```python
from build123d import *

# Parameters (mm, degrees)
F1_DEPTH = 2


with BuildPart() as f1:
    # F0 (on Top) → F1 (new body)
    with BuildSketch(Plane.XY):
        with BuildLine():
            Line((12, 38), (0, 38))
            Line((0, 38), (-12, 38))
            ThreePointArc((-12, 38), (-19.071081, 35.071055), (-22, 27.999963))
            Line((-22, 27.999963), (-22, 21.999963))
            ThreePointArc((-22, 21.999963), (-23.171507, 19.171602), (-25.999815, 17.999963))
            Line((-25.999815, 17.999963), (-28.499815, 17.999963))
            Line((-28.499815, 17.999963), (-28.499815, -7.000037))
            Line((-28.499815, -7.000037), (-25.999815, -7.000037))
            ThreePointArc((-25.999815, -7.000037), (-9.507625, -19.877017), (-18, -39))
            Line((-18, -39), (-18, -42))
            Line((-18, -42), (0, -42))
            Line((0, -42), (18, -42))
            Line((18, -42), (18, -39))
            ThreePointArc((18, -39), (9.507625, -19.877017), (25.999815, -7.000037))
            Line((25.999815, -7.000037), (28.499815, -7.000037))
            Line((28.499815, -7.000037), (28.499815, 17.999963))
            Line((28.499815, 17.999963), (25.999815, 17.999963))
            ThreePointArc((25.999815, 17.999963), (23.171507, 19.171602), (22, 21.999963))
            Line((22, 21.999963), (22, 27.999963))
            ThreePointArc((22, 27.999963), (19.071081, 35.071055), (12, 38))
        make_face()
    extrude(amount=F1_DEPTH)


solid = f1.part
```
Read the model definition and answer for the solid it produces. Units are mm, in the model's axes. A direction names the side the tool comes from. Coordinates: 2 decimals unless noted, no trailing zeros. Write each loop counter-clockwise with the first axis right and the second up, starting at its lowest first coordinate (ties: lowest second). Pieces come first, ordered by that corner, then holes. Notation, with made-up numbers: (50.25, 62) -> (96.25, 62) arc R22 ccw to (96.25, 98) -> close; hole circle Ø3 at (88, 89). An arc over 180 degrees is marked (long way). Return JSON: item names as keys, results as strings.
1. A cutting plane is placed at D-D (x = 10). Determine the outline of the cut face in (y, z).
Found:
{"outline": "(-42, 0) -> (-29.74, 0) -> (-29.74, 2) -> (-42, 2) -> close; (-18.26, 0) -> (38, 0) -> (38, 2) -> (-18.26, 2) -> close"}
2. A cutting plane is placed at C-C (y = -22). Determine the outline of the cut face in (x, z), and give its area (3 significant figures).
Found:
{"outline": "(-9.12, 0) -> (9.12, 0) -> (9.12, 2) -> (-9.12, 2) -> close", "area": "36.5 mm2"}
3. Each of these flat-tipped pins is pushed along its axis until it touches: P1, Ø1, axis at x = -27.5, z = 1, coming from the -Y side; P2, Ø1, axis at y = 24, z = 0.5, coming from the +X side; P3, Ø0.6, axis at y = -41, z = 1, coming from the -X side. Where does it stop, or does it pass through?
Found:
{"P1": "y = -7", "P2": "x = 22", "P3": "x = -18"}
4. A cutting plane is placed at A-A (z = 0.8). Determine the outline of the cut face in (x, y).
Found:
{"outline": "(-28.5, -7) -> (-26, -7) arc R17 cw to (-18, -39) -> (-18, -42) -> (18, -42) -> (18, -39) arc R17 cw to (26, -7) -> (28.5, -7) -> (28.5, 18) -> (26, 18) arc R4 cw to (22, 22) -> (22, 28) arc R10 ccw to (12, 38) -> (-12, 38) arc R10 ccw to (-22, 28) -> (-22, 22) arc R4 cw to (-26, 18) -> (-28.5, 18) -> close"}
5. Find the intervals of material crossed by line 1 along X through (y, z) = (24, 0.5); line 2 along Y through (x, z) = (-13.5, 0.25); line 3 along Y through (x, z) = (-17, 1.05), in increasing order. Write a range as from..to.
Found:
{"line 1": "-22..22", "line 2": "-42..-35.52, -12.48..37.89", "line 3": "-42..-38.42, -9.58..36.66"}
6. A cutting plane is placed at B-B (x = -16). Determine the outline of the cut face in (y, z).
Found:
{"outline": "(-42, 0) -> (-37.75, 0) -> (-37.75, 2) -> (-42, 2) -> close; (-10.25, 0) -> (37.17, 0) -> (37.17, 2) -> (-10.25, 2) -> close"}
7. A tool of negligible diameter and unlimited length cuts with its end or side. For faces 5 (the face through (9.434, -20.184, 0.986)), 6 (the face through (-27, 18, 1)), 7 (the face through (-18, -40, 1)), 8 (the face through (22, 25, 1)), from which of +Z, -Z, +X, -X, +Y, -Y can it reach the whole face along a straight path? Write none if from no direction.
Found:
{"face 5": "+Z, -Z, +X", "face 6": "+Z, -Z, -X, +Y", "face 7": "+Z, -Z, -X, -Y", "face 8": "+Z, -Z, +X, +Y"}
8. Determine the mould class of faces 1 (the face through (18, -41, 1)), 2 (the face through (-9.587, -19.572, 0.986)), 3 (the face through (27, -7, 1)), 4 (the face through (-18.99, 35.15, 0.99)) for opening direction Y: pulls with the +Y half, pulls with the -Y half, needs draft (parallel to the pull), parting line crosses it, or undercut.
Found:
{"face 1": "needs draft", "face 2": "undercut", "face 3": "pulls with the -Y half", "face 4": "pulls with the +Y half"}
